The listing builds one solid part. Answer for the finished solid, in the listing's coordinates (mm). Face numbers are marked on the shaded views. A direction names the side the tool comes from. Give positions to 0.01 mm unless a question says otherwise; leave off trailing zeros. Order: outer loops, then holes, each group sorted by start corner. A loop starts at its lowest first (then second) coordinate and runs counter-clockwise, first axis right, second up. Notation, with made-up numbers: (39, 12.5) - (90, 12.5) arc R23 ccw to (90, 22.5) - close; hole circle Ø4 at (33.25, 43.25). An arc over 180 degrees is marked (long way). Answer as a JSON object with one key per item and string values. Group by question number.
Q1. A cutting plane is placed at D-D, the plane z = -16. Give the vertices of the cut face in (x, y).
Q2. Consider line 1 (X direction, y = 13.85, z = -21.75); line 2 (X direction, y = 7, z = -3.5) (3 decimals); line 3 (Z direction, x = -45.5, y = 6.5). Determine where each line is inside the solid, lowest interval first.
Q3. Given pin 1 (1.5 mm diameter, centred on x = -23, z = -18.5, fed in from -Y); pin 2 (1.5 mm diameter, centred on y = 3, z = -9.5, fed in from +X); pin 3 (1.5 mm diameter, centred on x = -58.5, z = -30, fed in from -Y), each flat-ended and moving along its own axis, determine where each tip first touches the part or whether it passes through.
Q4. A cutting plane is placed at C-C, the plane x = -28.5. Give the vertices of the cut face in (y, z), and give its area (3 significant figures).
Q5. A cutting plane is placed at A-A, the plane z = -3.5. Give the vertices of the cut face in (x, y) (3 decimals), and give its area (3 significant figures).
Q6. For the marked faces 5, 6 and 7, determine the directions among +Z, -Z, +X, -X, +Y, -Y from which every point of the face is accessible in a straight line to the end or side of a thin tool.
Q7. The mould has two halves that part along X. Classify the marked faces 1, 2, 3 and 4: released by +X, released by -X, zero draft, split by the parting line, or undercut.
Q8. A cutting plane is placed at B-B, the plane x = -63. Give the vertices of the cut face in (y, z), and give its area (3 significant figures).
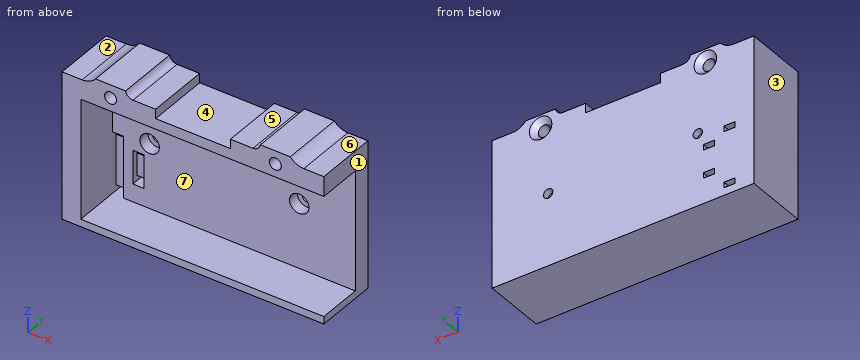
Autodesk Inventor part; units mm, degrees
ref_plane "YZ Plane" through (0, 0, 0) normal (1, 0, 0) x (0, 1, 0)
ref_plane "XZ Plane" through (0, 0, 0) normal (0, 1, 0) x (-1, 0, 0)
ref_plane "XY Plane" through (0, 0, 0) normal (0, 0, 1) x (1, 0, 0)
sketch "Эскиз1" plane through (0, 0, 0) normal (0, 1, 0) x (-1, 0, 0)
  line L0 (0, 0) -> (70, 0)
  line L1 (70, 0) -> (70, -41)
  line L2 (70, -41) -> (0, -41)
  line L3 (0, -41) -> (0, 0)
  line L4 (65, -7) -> (0, -7)
  line L5 (0, -7) -> (0, -39)
  line L6 (0, -39) -> (65, -39)
  line L7 (65, -39) -> (65, -7)
  line L8 (65, -7) -> (0, -39) construction
  line L9 (0, -7) -> (65, -39) construction
  line L10 (0, -7) -> (2, -7)
  point P0 (0, -7)
  dimension "d0" = 70
  dimension "d224" = 7
  dimension "d225" = 5
  dimension "d226" = 32
  dimension "d302" = 2
extrude "Выдавливание1" add sketch "Эскиз1" along normal blind 12 contours L0 L1 L2 L3 L6 L7 L4
sketch "Эскиз40" plane through (0, 12, 0) normal (0, 1, 0) x (1, 0, 0)
  line L0 (0, 41) -> (-70, 41)
  line L1 (0, 0) -> (-70, 0)
  line L2 (-70, 0) -> (-70, 41)
  line L3 (-70, 41) -> (0, 41)
  line L4 (0, 41) -> (0, 0)
  point P0 (0, 41)
extrude "Выдавливание32" add sketch "Эскиз40" along normal blind 4.8
sketch "Эскиз39" plane through (0, 16.8, 0) normal (0, 1, 0) x (1, 0, 0)
  line L0 (-70, 41) -> (-70, 0)
  line L1 (0, 41) -> (-70, 41)
  line L2 (0, 39) -> (0, 41)
  line L3 (-65, 39) -> (0, 39)
  line L4 (-65, 7) -> (-65, 39)
  line L5 (0, 7) -> (-65, 7)
  line L6 (0, 0) -> (0, 7)
  line L7 (-70, 0) -> (0, 0)
  line L8 (-70, 0) -> (0, 0) construction
  line L9 (-35, 0) -> (-35, 7) construction
  line L10 (-57.025, 3.5) -> (-12.975, 3.5) construction
  point P0 (-35, 3.5)
  dimension "d356" = 44.05
hole "Отверстие6" at (-12.975, 16.8, -3.5) at (-57.025, 16.8, -3.5) direction (0, -1, 0) diameter 3.2 end through all countersink diameter 6 countersink angle 90
sketch "Эскиз49" plane through (0, 12, 0) normal (0, 1, 0) x (1, 0, 0)
  line L0 (-70, 0) -> (0, 0) construction
  line L1 (-35, 0) -> (-35, 21.75) construction
  line L2 (-55, 21.75) -> (-15, 21.75) construction
  dimension "d369" = 21.75
  dimension "d370" = 40
hole "Отверстие8" at (-15, 12, -21.75) at (-55, 12, -21.75) direction (0, 1, 0) diameter 2.5 end through all counterbore diameter 5.2 counterbore depth 3
sketch "Эскиз48" plane through (0, 16.8, 0) normal (0, 1, 0) x (1, 0, 0)
  line L0 (-53.025, 0) -> (-16.975, 0)
  line L1 (-16.975, 0) -> (-16.975, 4.2)
  line L2 (-16.975, 4.2) -> (-53.025, 4.2)
  line L3 (-53.025, 4.2) -> (-53.025, 0)
  line L4 (-70, 0) -> (0, 0)
  line L5 (-70, 41) -> (-70, 0)
  line L6 (-70, 0) -> (-61.025, 0)
  line L7 (-61.025, 0) -> (-61.025, 1.7)
  line L8 (-61.025, 1.7) -> (-70, 1.7)
  line L9 (-70, 1.7) -> (-70, 0)
  line L10 (0, 0) -> (-8.975, 0)
  line L11 (-8.975, 0) -> (-8.975, 1.7)
  line L12 (-8.975, 1.7) -> (0, 1.7)
  line L13 (0, 1.7) -> (0, 0)
  line L14 (-61.025, 0) -> (-53.025, 0)
  line L15 (-53.025, 0) -> (-53.025, 7)
  line L16 (-53.025, 7) -> (-61.025, 7)
  line L17 (-61.025, 7) -> (-61.025, 0)
  circle A0 centre (-57.025, 3.5) radius 1.6
  line L18 (-61.025, 0) -> (-53.025, 7) construction
  line L19 (-53.025, 0) -> (-61.025, 7) construction
  line L20 (-8.975, 0) -> (-16.975, 0)
  line L21 (-16.975, 0) -> (-16.975, 7)
  line L22 (-16.975, 7) -> (-8.975, 7)
  line L23 (-8.975, 7) -> (-8.975, 0)
  circle A1 centre (-12.975, 3.5) radius 3
  line L24 (-8.975, 0) -> (-16.975, 7) construction
  line L25 (-16.975, 0) -> (-8.975, 7) construction
  line L26 (-53.025, 0) -> (-45, 0)
  line L27 (-45, 0) -> (-45, 1.7)
  line L28 (-45, 1.7) -> (-53.025, 1.7)
  line L29 (-53.025, 1.7) -> (-53.025, 0)
  line L30 (-16.975, 0) -> (-25, 0)
  line L31 (-25, 0) -> (-25, 1.7)
  line L32 (-25, 1.7) -> (-16.975, 1.7)
  line L33 (-16.975, 1.7) -> (-16.975, 0)
  line L34 (-45, 1.7) -> (-45, 4.2)
  line L35 (-25, 1.7) -> (-25, 4.2)
  point P0 (-35, 0)
  point P1 (-8.975, 0)
  point P2 (-53.025, 1.7)
  point P3 (-16.975, 1.7)
  dimension "d359" = 4.2
  dimension "d363" = 8
  dimension "d364" = 8
  dimension "d365" = 1.7
  dimension "d366" = 8.025
extrude "Выдавливание38" cut sketch "Эскиз48" against normal through all contours L3 L28 L27 L0 | L27 L34 L2 L35 L31 L0 | L4 L5 L8 L7 | L31 L32 L1 L0 | L11 L12 L13 L4
fillet "Сопряжение2" radius 2 2 edges at (-16.975, 8.4, -1.7) (-53.025, 8.4, -1.7)
fillet "Сопряжение2" radius 4.7 2 edges at (-8.975, 8.4, -1.7) (-61.025, 8.4, -1.7)
sketch "Эскиз50" plane through (0, 16.8, 0) normal (0, 1, 0) x (1, 0, 0)
  line L0 (-62, 22.5) -> (-62, 24)
  line L1 (-62, 24) -> (-65, 24)
  line L2 (-65, 24) -> (-65, 22.5)
  line L3 (-65, 22.5) -> (-62, 22.5)
  line L4 (-62, 37.5) -> (-62, 39)
  line L5 (-62, 39) -> (-65, 39)
  line L6 (-65, 39) -> (-65, 37.5)
  line L7 (-65, 37.5) -> (-62, 37.5)
  line L8 (-70, 41) -> (-70, 1.7)
  line L9 (0, 41) -> (-70, 41)
  line L10 (-63.5, 24) -> (-63.5, 37.5) construction
  line L11 (-63.5, 30.75) -> (-58, 30.75) construction
  line L12 (-58, 30.75) -> (-58, 26.75) construction
  line L13 (-59.5, 25.25) -> (-56.5, 25.25)
  line L14 (-56.5, 25.25) -> (-56.5, 26.75)
  line L15 (-56.5, 26.75) -> (-59.5, 26.75)
  line L16 (-59.5, 26.75) -> (-59.5, 25.25)
  line L17 (-59.5, 32.75) -> (-56.5, 32.75)
  line L18 (-56.5, 32.75) -> (-56.5, 34.25)
  line L19 (-56.5, 34.25) -> (-59.5, 34.25)
  line L20 (-59.5, 34.25) -> (-59.5, 32.75)
  point P0 (0, 0)
  dimension "d378" = 13.5
  dimension "d379" = 1.5
  dimension "d380" = 3
  dimension "d385" = 5
  dimension "d386" = 2
  dimension "d389" = 6
  dimension "d390" = 4
  dimension "d391" = 5.5
extrude "Выдавливание39" cut sketch "Эскиз50" against normal through all
sketch "Эскиз51" plane through (0, 12, 0) normal (0, -1, 0) x (1, 0, 0)
  line L0 (-62, -24) -> (-65, -24)
  line L1 (-65, -37.5) -> (-62, -37.5)
  line L2 (-62, -24) -> (-65, -24)
  line L3 (-65, -24) -> (-65, -37.5)
  line L4 (-65, -37.5) -> (-62, -37.5)
  line L5 (-62, -37.5) -> (-62, -24)
  line L6 (-56.5, -26.75) -> (-59.5, -26.75)
  line L7 (-59.5, -32.75) -> (-56.5, -32.75)
  line L8 (-59.5, -26.75) -> (-56.5, -26.75)
  line L9 (-56.5, -26.75) -> (-56.5, -32.75)
  line L10 (-56.5, -32.75) -> (-59.5, -32.75)
  line L11 (-59.5, -32.75) -> (-59.5, -26.75)
  point P0 (0, 0)
extrude "Выдавливание40" cut sketch "Эскиз51" against normal blind 1.5
properties part number "Стойка под электроннику"
Reply:
{
 "1": {"outline": "(-70, 0) - (-65, 0) - (-65, 12) - (0, 12) - (0, 16.8) - (-70, 16.8) - close"},
 "2": {"line 1": "x = -70 to -57.6, -52.4 to -17.6, -12.4 to 0", "line 2": "x = -70 to -58.625, -55.425 to -45, -25 to -14.575, -11.375 to 0", "line 3": "z = -41 to -39, -7 to -1.7"},
 "3": {"pin 1": "stops at y = 12", "pin 2": "stops at x = -65", "pin 3": "stops at y = 13.5"},
 "4": {"outline": "(0, -41) - (16.8, -41) - (16.8, -4.2) - (0, -4.2) - (0, -7) - (12, -7) - (12, -39) - (0, -39) - close", "area": "234 mm^2"},
 "5": {"outline": "(-70, 0) - (-58.625, 0) - (-58.625, 15.4) - (-60.025, 16.8) - (-70, 16.8) - close; (-55.425, 0) - (-45, 0) - (-45, 16.8) - (-54.025, 16.8) - (-55.425, 15.4) - close; (-25, 0) - (-14.575, 0) - (-14.575, 15.4) - (-15.975, 16.8) - (-25, 16.8) - close; (-11.375, 0) - (0, 0) - (0, 16.8) - (-9.975, 16.8) - (-11.375, 15.4) - close", "area": "729 mm^2"},
 "6": {"face 5": "+Z, +Y, -Y", "face 6": "+Z, +X, +Y, -Y", "face 7": "+X, -Y"},
 "7": {"face 1": "released by +X", "face 2": "zero draft", "face 3": "released by -X", "face 4": "undercut"},
 "8": {"outline": "(0, -41) - (16.8, -41) - (16.8, -39) - (0, -39) - close; (0, -7) - (12, -7) - (12, -22.5) - (16.8, -22.5) - (16.8, -1.4) - (0, -1.4) - close; (13.5, -37.5) - (16.8, -37.5) - (16.8, -24) - (13.5, -24) - close", "area": "247 mm^2"}
}
